Geometry: see drawing. Coordinates: mm, zero at the bounding-box minimum. A direction names the side the tool comes from. Give positions to 0.01 mm unless a question says otherwise; leave off trailing zeros. Write each loop counter-clockwise with the first axis right and the second up, starting at its lowest first coordinate (ties: lowest second). Pieces come first, ordered by that corner, then holes. Notation, with made-up numbers: (80.5, 75) - (136.5, 75) arc R23 ccw to (136.5, 109) - close; hole circle Ø9 at (64.25, 16.5). An arc over 180 degrees is marked (long way). One line per question, with ' | ' between items. Start each with the question number.
(1) Section A-A, the plane y = 10. Return loops of the section in (x, z), plus the area to 3 significant figures.
(2) Ray query, line 1 (Y direction, x = 5, z = 2.1); line 2 (Y direction, x = 39.4, z = 10); line 3 (X direction, y = 7, z = 7.5). Return the intervals inside material, ascending. Write a range as [from, to].
(3) Draft query along X for the marked faces 1, 2 and 3. Return one class per face: +X half, -X half, draft (parallel to the pull), parting line (faces both ways), or undercut.
(4) Pin query (flat end, axial travel): pin 1 (5 mm diameter, centred on y = 7.5, z = 10.5, fed in from -X); pin 2 (8 mm diameter, centred on x = 35, z = 11.5, fed in from +Y); pin 3 (2.5 mm diameter, centred on x = 40, z = 12, fed in from -Y). Return the tip coordinate at first contact, or that it passes through.
(5) Access query for the marked faces 4, 5 and 6. Directions: +Z, -Z, +X, -X, +Y, -Y. A direction counts if a zero-diameter tool reaches every point of the face in a straight line with its end or side. Return the directions, or none.
(6) Section D-D, the plane z = 10. Return loops of the section in (x, y), plus the area to 3 significant figures.
(7) Section C-C, the plane z = 13.75. Return loops of the section in (x, y), plus the area to 3 significant figures.
(8) Section B-B, the plane x = 21.5. Return loops of the section in (y, z).
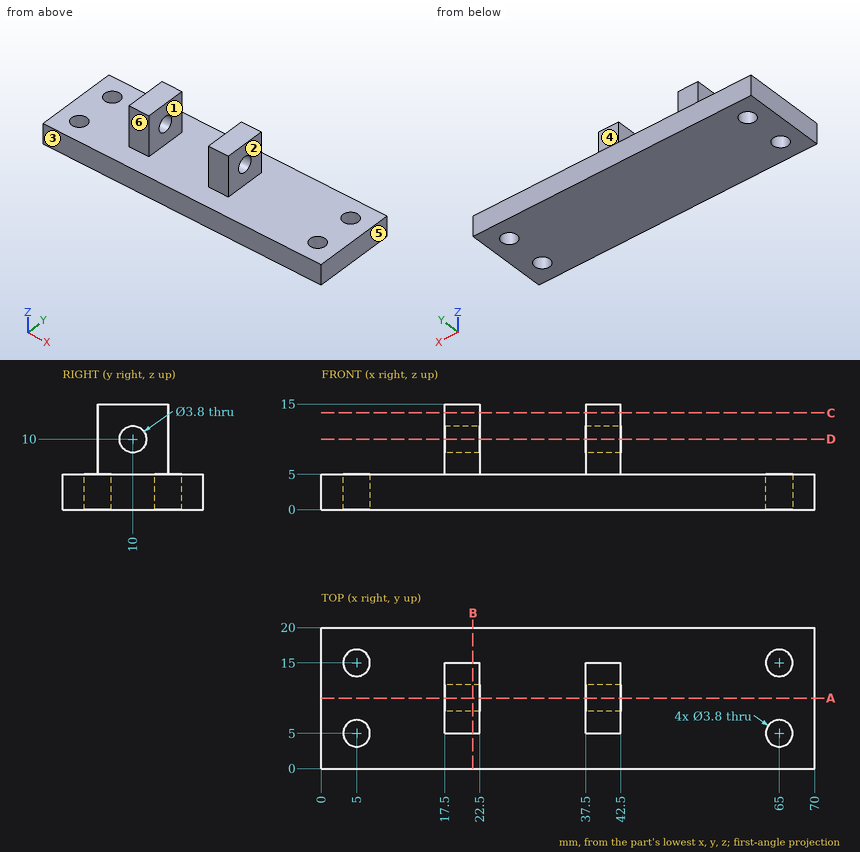
Check sheet entries:
1) outline: (0, 0) - (70, 0) - (70, 5) - (42.5, 5) - (42.5, 8.1) - (37.5, 8.1) - (37.5, 5) - (22.5, 5) - (22.5, 8.1) - (17.5, 8.1) - (17.5, 5) - (0, 5) - close; (17.5, 11.9) - (22.5, 11.9) - (22.5, 15) - (17.5, 15) - close; (37.5, 11.9) - (42.5, 11.9) - (42.5, 15) - (37.5, 15) - close | area: 412 mm²
2) line 1: [0, 3.1], [6.9, 13.1], [16.9, 20] | line 2: [5, 8.1], [11.9, 15] | line 3: [17.5, 22.5], [37.5, 42.5]
3) face 1: undercut | face 2: +X half | face 3: draft
4) pin 1: x = 17.5 | pin 2: y = 15 | pin 3: y = 5
5) face 4: +Z, +X, -X, +Y | face 5: +Z, -Z, +X, +Y, -Y | face 6: +Z, +X, -X, -Y
6) outline: (17.5, 5) - (22.5, 5) - (22.5, 8.1) - (17.5, 8.1) - close; (17.5, 11.9) - (22.5, 11.9) - (22.5, 15) - (17.5, 15) - close; (37.5, 5) - (42.5, 5) - (42.5, 8.1) - (37.5, 8.1) - close; (37.5, 11.9) - (42.5, 11.9) - (42.5, 15) - (37.5, 15) - close | area: 62.0 mm²
7) outline: (17.5, 5) - (22.5, 5) - (22.5, 15) - (17.5, 15) - close; (37.5, 5) - (42.5, 5) - (42.5, 15) - (37.5, 15) - close | area: 100 mm²
8) outline: (0, 0) - (20, 0) - (20, 5) - (15, 5) - (15, 15) - (5, 15) - (5, 5) - (0, 5) - close; hole circle Ø3.8 at (10, 10)
